Verification items for the finished model (mm, model axes). A direction names the side the tool comes from. Give positions to 0.01 mm unless a question says otherwise; leave off trailing zeros. Order: outer loops, then holes, each group sorted by start corner. A loop starts at its lowest first (then second) coordinate and runs counter-clockwise, first axis right, second up.
from build123d import *

# Parameters (mm, degrees)
CYLINDER034_R     = 3
CYLINDER034_DEPTH = 3.6
CYLINDER035_R     = 1.5
CYLINDER035_DEPTH = 14


with BuildPart() as cylinder034:
    # Cylinder034 → Cylinder034 (new body)
    with BuildSketch(Plane.XY.offset(10)):
        Circle(CYLINDER034_R)
    extrude(amount=CYLINDER034_DEPTH)


with BuildPart() as obj1:
    # Cylinder035 → Cylinder035 (new body)
    with BuildSketch(Plane.XY.offset(10)):
        Circle(CYLINDER035_R)
    extrude(amount=CYLINDER035_DEPTH)

    # Fusion007002009027003005008003003018004: union Cylinder034
    add(cylinder034.part)


with BuildPart() as obj1_1:
    # Fusion007002009027003005008003003018004 placement: moved
    add(obj1.part.moved(Location((128, 14, -137))))


solid = obj1_1.part
(1) Section check A-A, the plane x = 128. Enter the section's corners in (y, z).
Solved:
outline: (11, -127) - (17, -127) - (17, -123.4) - (15.5, -123.4) - (15.5, -113) - (12.5, -113) - (12.5, -123.4) - (11, -123.4) - close
(2) Set-up check for faces 1 (the flat face through (128, 14, -113)), 2 (the cylindrical face through (126.5, 14.07, -118.27)): record each of +Z, -Z, +X, -X, +Y, -Y from which the full face is reachable in a straight line by a thin tool's end or side.
Solved:
face 1: +Z, +X, -X, +Y, -Y
face 2: +Z
(3) Section check B-B, the plane y = 14. Enter the section's corners in (x, z), then the cut area to 3 significant figures.
Solved:
outline: (125, -127) - (131, -127) - (131, -123.4) - (129.5, -123.4) - (129.5, -113) - (126.5, -113) - (126.5, -123.4) - (125, -123.4) - close
area: 52.8 mm2
(4) Section check D-D, the plane y = 12.05. Enter the section's corners in (x, z), then the cut area to 3 significant figures.
Solved:
outline: (125.72, -127) - (130.28, -127) - (130.28, -123.4) - (125.72, -123.4) - close
area: 16.4 mm2
(5) Scan lines: line 1 (Z direction, x = 129.75, y = 16.15); line 2 (X direction, y = 14.1, z = -114.5); line 3 (Y direction, x = 127.9, z = -126.5). Record each from-to range of solid material in increasing order.
Solved:
line 1: z = -127 to -123.4
line 2: x = 126.5 to 129.5
line 3: y = 11 to 17
(6) Section check C-C, the plane z = -125. Enter the section's corners in (x, y), then the cut area to 3 significant figures.
Solved:
outline: circle Ø6 at (128, 14)
area: 28.3 mm2
(7) Go/stop test with flat-tipped pins: pin 1 (1 mm diameter, centred on y = 16.5, z = -119.5, fed in from -X); pin 2 (3 mm diameter, centred on x = 126.5, z = -120, fed in from +Y). Record where each tip stops, or that it passes through.
Solved:
pin 1: passes through
pin 2: stops at y = 15.5
